```python
from build123d import *

# Parameters (mm, degrees)
SKETCH1_W          = 304.8
SKETCH1_H          = 152.4
EXTRUDE1_DEPTH     = 12.7
SKETCH2_W          = 12.7
SKETCH2_H          = 19.05
EXTRUDE2_DEPTH     = 171.861025398
SKETCH3_R          = 1.5875
CUT_EXTRUDE1_DEPTH = 171.861025398


with BuildPart() as part:
    # Sketch1 → Extrude1 (new body)
    with BuildSketch(Plane(origin=(0, 0, 0), x_dir=(1, 0, 0), z_dir=(0, 1, 0))):
        Rectangle(SKETCH1_W, SKETCH1_H)
    extrude(amount=EXTRUDE1_DEPTH)

    # Sketch2 → Extrude2 (cut, through all)
    with BuildSketch(Plane(origin=(0, 12.7, 0), x_dir=(1, 0, 0), z_dir=(0, 1, 0))):
        with Locations((-48.895, 44.45)):
            Rectangle(SKETCH2_W, SKETCH2_H)
        with Locations((48.895, 44.45)):
            Rectangle(SKETCH2_W, SKETCH2_H)
        with Locations((-48.895, -44.45)):
            Rectangle(SKETCH2_W, SKETCH2_H)
        with Locations((48.895, -44.45)):
            Rectangle(SKETCH2_W, SKETCH2_H)
        with Locations((146.05, 44.45)):
            Rectangle(SKETCH2_W, SKETCH2_H)
        with Locations((-146.05, 44.45)):
            Rectangle(SKETCH2_W, SKETCH2_H)
        with Locations((146.05, -44.45)):
            Rectangle(SKETCH2_W, SKETCH2_H)
        with Locations((-146.05, -44.45)):
            Rectangle(SKETCH2_W, SKETCH2_H)
    extrude(amount=-EXTRUDE2_DEPTH, mode=Mode.SUBTRACT)

    # Sketch3 → Cut-Extrude1 (cut, through all)
    with BuildSketch(Plane.XZ):
        with Locations(Location((31.6865, 36.796180661, 0), (0, 0, 270))):
            Circle(SKETCH3_R)
        with Locations(Location((31.6865, -26.703819339, 0), (0, 0, 270))):
            Circle(SKETCH3_R)
        with Locations(Location((-31.6865, -26.703819339, 0), (0, 0, 90))):
            Circle(SKETCH3_R)
        with Locations(Location((-31.6865, 36.796180661, 0), (0, 0, 90))):
            Circle(SKETCH3_R)
    extrude(amount=-CUT_EXTRUDE1_DEPTH, mode=Mode.SUBTRACT)


solid = part.part
```
Can you work these out from the model? Positions are in its coordinate system, mm. A direction names the side the tool comes from. Round coordinates to 2 decimals unless told otherwise and drop trailing zeros. Loops run counter-clockwise (first coordinate to the right, second up) from the corner with the lowest first, then second, coordinate; pieces in that order, holes last. Notation, with made-up numbers: (10, 7.25) -> (44, 7.25) arc R28 ccw to (44, 39.25) -> close; hole circle Ø1 at (-22.5, 30.25). An arc over 180 degrees is marked (long way). One line per item, written item: value. Start each with the question number.
1. If I drill on probe 1 along Z at (x, y) = (46, 9) (3 decimals); probe 2 along X at (y, z) = (4.75, -38) (3 decimals), over which ranges is the centre line in solid material (lowest first)?
2. If we section it at A-A, the plane z = -51: Write out the boundary of the cut face in (x, y) (3 decimals), then the cut area to 3 significant figures.
3. For faces 1 (the flat face through (146, 6, 53.975)), 2 (the flat face through (-49, 6, 34.925)), 3 (the flat face through (-152.4, 6, 65)), 4 (the flat face through (-139.7, 6, 45)), which set-ups out of +Z, -Z, +X, -X, +Y, -Y let a thin tool reach every point of the face, with its end or its side?
4. For pin 1 (6.5 mm diameter, centred on y = 4.5, z = -49, fed in from +X); pin 2 (1.5 mm diameter, centred on x = -62.5, z = 58, fed in from -Y); pin 3 (3 mm diameter, centred on x = 31.69, z = -26.7, fed in from -Y), each with a flat end and sliding along its axis, tell me the tip position at first contact or that it passes through.
5. If we mould it in two halves opening along X, with no side actions, what happens to faces 5 (the flat face through (49, 6, -53.975)), 6 (the flat face through (152.4, 6, -65)), 7 (the flat face through (-139.7, 6, -44)), 8 (the flat face through (-42.545, 6, -44))? For each: pulls with the +X half, pulls with the -X half, needs draft (parallel to the pull), parting line crosses it, or undercut.
6. If we section it at B-B, the plane y = 10: Give the number of separate pieces and of enclosed holes in the cut face, then the cut area to 3 significant figures.
Calculated:
1. probe 1: z = -76.2 to -53.975, -34.925 to 34.925, 53.975 to 76.2
1. probe 2: x = -139.7 to -55.245, -42.545 to 42.545, 55.245 to 139.7
2. outline: (-139.7, 0) -> (-55.245, 0) -> (-55.245, 12.7) -> (-139.7, 12.7) -> close; (-42.545, 0) -> (42.545, 0) -> (42.545, 12.7) -> (-42.545, 12.7) -> close; (55.245, 0) -> (139.7, 0) -> (139.7, 12.7) -> (55.245, 12.7) -> close
2. area: 3,230 mm²
3. face 1: +X, +Y, -Y
3. face 2: +Y, -Y
3. face 3: +Z, -Z, -X, +Y, -Y
3. face 4: -X, +Y, -Y
4. pin 1: stops at x = 139.7
4. pin 2: stops at y = 0
4. pin 3: passes through
5. face 5: undercut
5. face 6: pulls with the +X half
5. face 7: pulls with the -X half
5. face 8: undercut
6. separate pieces: 1
6. enclosed holes: 8
6. area: 44,500 mm²
